Geometry: final body of the model. Coordinates: model frame, mm. A direction names the side the tool comes from. Coordinates: 2 decimals unless noted, no trailing zeros. Order: outer loops, then holes, each group sorted by start corner. A loop starts at its lowest first (then second) coordinate and runs counter-clockwise, first axis right, second up. Notation, with made-up numbers: M -6,42 L 41,42 A8 cw 41,48 Z; hole C 66,-32 d4. An arc over 180 degrees is marked long. Use CSV: the item, a comma, the result in double quotes. Start each with the question number.
Q1. Access query for faces 1 (the face through (0, 0, 3)), 2 (the face through (-6.7, 2.98, 1.52)), 3 (the face through (0, 0, 0)), 4 (the face through (-7, 0, 1)), 5 (the face through (15.4, -0.34, 4.63)). Directions: +Z, -Z, +X, -X, +Y, -Y. A direction counts if a zero-diameter tool reaches every point of the face in a straight line with its end or side. Return the directions, or none.
Q2. Section query A-A, the plane y = 0.5. Output: boundary loops of the cut face in (x, z).
Q3. Section query C-C, the plane x = 3.75. Output: boundary loops of the cut face in (y, z).
Q4. Ray query, probe 1 along Z at (x, y) = (-3, -2); probe 2 along X at (y, z) = (0.75, 0.75); probe 3 along X at (y, z) = (-0.75, 4.25). Return the intervals inside material, ascending.
Q5. Section query D-D, the plane z = -1. Output: boundary loops of the cut face in (x, y), and give its area (3 significant figures).
Q6. First-contact query: P1, Ø1.5, axis at x = 3.5, y = 2, coming from the -Z side; P2, Ø2.5, axis at x = -4.72, y = 0, coming from the +Z side; P3, Ø1, axis at x = 20, z = 1, coming from the +Y side. Flat tips, straight axial feed; report the tip coordinate or a pass-through.
Q7. Section query B-B, the plane z = 2.25. Output: boundary loops of the cut face in (x, y).
Autodesk Inventor part; units mm, degrees
ref_plane "YZ Plane" through (0, 0, 0) normal (1, 0, 0) x (0, 1, 0)
ref_plane "XZ Plane" through (0, 0, 0) normal (0, 1, 0) x (-1, 0, 0)
sketch "Sketch1" plane through (0, 0, 0) normal (0, 0, 1) x (1, 0, 0)
  line L0 (-7, -0.2342) -> (-7, 3.2658)
  line L1 (-7, 3.2658) -> (8, 3.2658)
  line L2 (8, 3.2658) -> (8, -3.7342)
  line L3 (8, -3.7342) -> (-7, -3.7342)
  line L4 (-7, -3.7342) -> (-7, -0.2342)
  point P0 (0, 0)
  dimension "d0" = 15
  dimension "d1" = 15
  dimension "d2" = 7
  dimension "d3" = 3.5
  dimension "d4" = 7
extrude "Extrusion1" add sketch "Sketch1" along normal blind 3
fillet "Fillet1" radius 1 1 edges at (8, 3.2658, 1.5)
fillet "Fillet2" radius 1 1 edges at (8, -3.7342, 1.5)
fillet "Fillet3" radius 1 2 edges at (-7, 3.2658, 1.5) (-7, -3.7342, 1.5)
sketch "Sketch2" plane through (0, 0, 3) normal (0, 0, 1) x (1, 0, 0)
  circle A0 centre (-4.7192, 0) radius 0.9993
  point P0 (0, 0)
extrude "Extrusion2" cut sketch "Sketch2" against normal blind 3
sketch "Sketch3" plane through (8, 2.2658, 3) normal (1, 0, 0) x (0, 0, -1)
  circle A0 centre (1.5431, -2.4625) radius 3.1761
  point P0 (3, -2.2658)
extrude "Extrusion3" add sketch "Sketch3" along normal blind 15
sketch "Sketch4" plane through (23, -0.1967, 1.4569) normal (1, 0, 0) x (0, 0, -1)
  point P0 (1.4569, 0.1967)
sketch "Sketch5" plane through (0, 0, 0) normal (0, 0, 1) x (1, 0, 0)
  point P0 (0, 0)
thread "Thread1"
properties part number "end factor"
Responses:
1,face 1,"+Z, -X, +Y, -Y"
1,face 2,"+Z, -Z, -X, +Y"
1,face 3,"-Z, -X, +Y, -Y"
1,face 4,"+Z, -Z, -X, +Y, -Y"
1,face 5,"+X"
2,outline,"M -7,0 L -5.58,0 L -5.58,3 L -7,3 Z; M -3.85,0 L 8,0 L 8,-1.64 L 23,-1.64 L 23,4.56 L 8,4.56 L 8,3 L -3.85,3 Z"
3,outline,"M -3.73,0 L 3.27,0 L 3.27,3 L -3.73,3 Z"
4,probe 1,"z = 0 to 3"
4,probe 2,"x = -7 to -5.38, -4.06 to 23"
4,probe 3,"x = 8 to 23"
5,outline,"M 8,-2.21 L 23,-2.21 L 23,1.82 L 8,1.82 Z"
5,area,"60.4 mm²"
6,P1,"stops at z = 0"
6,P2,"stops at z = 3"
6,P3,"stops at y = 2.98"
7,outline,"M -7,-2.73 A1 ccw -6,-3.73 L 7,-3.73 A1 ccw 8,-2.73 L 8,-3.27 L 23,-3.27 L 23,2.88 L 8,2.88 L 8,2.27 A1 ccw 7,3.27 L -6,3.27 A1 ccw -7,2.27 Z; hole C -4.72,0 d2"
